```python
from build123d import *

# Parameters (mm, degrees)
SKETCH_1_W          = 23
SKETCH_1_H          = 10.8
EXTRUDE_1_DEPTH     = 34
CUT_EXTRUDE_1_DEPTH = 35
SKETCH_3_W          = 7
SKETCH_3_H          = 22
EXTRUDE_2_DEPTH     = 9
EXTRUDE_3_DEPTH     = 22
SKETCH_7_R          = 3.25
CUT_EXTRUDE_7_DEPTH = 1
CUT_EXTRUDE_8_REACH = 11.8
SKETCH_8_R          = 1.5


with BuildPart() as part:
    # 草图1 → 凸台-拉伸1 (new body)
    with BuildSketch(Plane(origin=(0, 0, 0), x_dir=(1, 0, 0), z_dir=(0, 1, 0))):
        Rectangle(SKETCH_1_W, SKETCH_1_H)
    extrude(amount=EXTRUDE_1_DEPTH)

    # 草图2 → 切除-拉伸1 (cut, through all)
    with BuildSketch(Plane(origin=(0, 34, 0), x_dir=(1, 0, 0), z_dir=(0, 1, 0))):
        Polygon((-6.5, 1.4), (6.5, 1.4), (6.5, -2.4), (3.15, -2.4), (3.15, -5.4), (-3.15, -5.4), (-3.15, -2.4), (-6.5, -2.4), align=None)
    extrude(amount=-CUT_EXTRUDE_1_DEPTH, mode=Mode.SUBTRACT)

    # 草图3 → 凸台-拉伸2 (add)
    with BuildSketch(Plane(origin=(0, 0, -5.4), x_dir=(-1, 0, 0), z_dir=(0, 0, -1))):
        with Locations((-10, 17)):
            Rectangle(SKETCH_3_W, SKETCH_3_H)
        with Locations((10, 17)):
            Rectangle(SKETCH_3_W, SKETCH_3_H)
    extrude(amount=-EXTRUDE_2_DEPTH)

    # 草图5 → 凸台-拉伸3 (add)
    with BuildSketch(Plane.XZ.offset(-6)):
        Polygon((11.5, 5.4), (11.5, 3.6), (13.5, 3.6), align=None)
        Polygon((-13.5, 3.6), (-11.5, 5.4), (-11.5, 3.6), align=None)
    extrude(amount=-EXTRUDE_3_DEPTH)

    # 草图7 → 切除-拉伸7 (cut)
    with BuildSketch(Plane.XY.offset(5.4)):
        with Locations((-10, 24.5)):
            Circle(SKETCH_7_R)
        with Locations((-10, 9.5)):
            Circle(SKETCH_7_R)
        with Locations((10, 9.5)):
            Circle(SKETCH_7_R)
        with Locations((10, 24.5)):
            Circle(SKETCH_7_R)
    extrude(amount=-CUT_EXTRUDE_7_DEPTH, mode=Mode.SUBTRACT)

    # 草图8 → 切除-拉伸8 (cut, up to next)
    with BuildSketch(Plane.XY.offset(4.4), mode=Mode.PRIVATE) as cut_extrude_8_sk1:
        with Locations((-10, 24.5)):
            Circle(SKETCH_8_R)
    cut_extrude_8_tool1 = extrude(cut_extrude_8_sk1.sketch, amount=-CUT_EXTRUDE_8_REACH, mode=Mode.PRIVATE) & part.part
    add(cut_extrude_8_tool1.solids().sort_by_distance((-10, 24.5, 4.4))[0], mode=Mode.SUBTRACT)
    # 草图8 → 切除-拉伸8 (cut, up to next)
    with BuildSketch(Plane.XY.offset(4.4), mode=Mode.PRIVATE) as cut_extrude_8_sk2:
        with Locations((10, 24.5)):
            Circle(SKETCH_8_R)
    cut_extrude_8_tool2 = extrude(cut_extrude_8_sk2.sketch, amount=-CUT_EXTRUDE_8_REACH, mode=Mode.PRIVATE) & part.part
    add(cut_extrude_8_tool2.solids().sort_by_distance((10, 24.5, 4.4))[0], mode=Mode.SUBTRACT)
    # 草图8 → 切除-拉伸8 (cut, up to next)
    with BuildSketch(Plane.XY.offset(4.4), mode=Mode.PRIVATE) as cut_extrude_8_sk3:
        with Locations((-10, 9.5)):
            Circle(SKETCH_8_R)
    cut_extrude_8_tool3 = extrude(cut_extrude_8_sk3.sketch, amount=-CUT_EXTRUDE_8_REACH, mode=Mode.PRIVATE) & part.part
    add(cut_extrude_8_tool3.solids().sort_by_distance((-10, 9.5, 4.4))[0], mode=Mode.SUBTRACT)
    # 草图8 → 切除-拉伸8 (cut, up to next)
    with BuildSketch(Plane.XY.offset(4.4), mode=Mode.PRIVATE) as cut_extrude_8_sk4:
        with Locations((10, 9.5)):
            Circle(SKETCH_8_R)
    cut_extrude_8_tool4 = extrude(cut_extrude_8_sk4.sketch, amount=-CUT_EXTRUDE_8_REACH, mode=Mode.PRIVATE) & part.part
    add(cut_extrude_8_tool4.solids().sort_by_distance((10, 9.5, 4.4))[0], mode=Mode.SUBTRACT)


solid = part.part
```
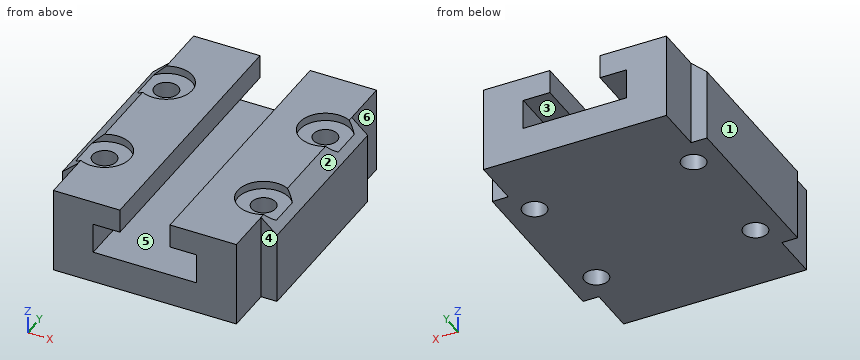
The listing builds one solid part. Answer for the finished solid, in the listing's coordinates (mm). Face numbers are marked on the shaded views. A direction names the side the tool comes from. Give positions to 0.01 mm unless a question says otherwise; leave off trailing zeros. Order: outer loops, then holes, each group sorted by start corner. A loop starts at its lowest first (then second) coordinate and runs counter-clockwise, first axis right, second up. Notation, with made-up numbers: (12.25, 1) -> (49.25, 1) arc R17 ccw to (49.25, 19) -> close; hole circle Ø8 at (32, 47.5). An arc over 180 degrees is marked (long way). Answer as a JSON object with one key per item and string values. Group by question number.
Item 1: The part is cut by section D-D on x = 5.75. Write down the section's boundary in (y, z).
Item 2: The part is cut by section B-B on z = -0.25. Write down the section's boundary in (x, y).
Item 3: Determine the mould class of the marked faces 1, 2 and 3 for opening direction Z: pulls with the +Z half, pulls with the -Z half, needs draft (parallel to the pull), parting line crosses it, or undercut.
Item 4: A tool of negligible diameter and unlimited length cuts with its end or side. For the marked faces 4, 5 and 6, from which of +Z, -Z, +X, -X, +Y, -Y can it reach the whole face along a straight path? Write none if from no direction.
Item 5: Flat-ended cylindrical pins translate along their axes: pin 1 (6.5 mm diameter, centred on x = -1.5, y = 9.5, fed in from +Z); pin 2 (4.5 mm diameter, centred on x = -10.5, y = 25, fed in from +Z); pin 3 (2.5 mm diameter, centred on x = 10, y = 24.5, fed in from +Z); pin 4 (1.8 mm diameter, centred on y = 1.5, z = 2.5, fed in from -X). Find the tip coordinate at first contact, or state that the pin passes through.
Item 6: The part is cut by section A-A on x = 10. Write down the section's boundary in (y, z), and give its area (3 significant figures).
Item 7: Consider L1, parallel to Y at x = -10, z = 5; L2, parallel to Y at x = -10, z = 2.75; L3, parallel to Z at x = -5.25, y = 26. Determine where each line is inside the solid, lowest interval first. Write a range as from..to.
Item 8: The part is cut by section C-C on y = 24.5. Write down the section's boundary in (x, z), and give its area (3 significant figures).
Result set:
{
 "1": {"outline": "(0, -5.4) -> (34, -5.4) -> (34, -1.4) -> (0, -1.4) -> close; (0, 2.4) -> (34, 2.4) -> (34, 5.4) -> (0, 5.4) -> close"},
 "2": {"outline": "(-13.5, 6) -> (-11.5, 6) -> (-11.5, 0) -> (-6.5, 0) -> (-6.5, 34) -> (-11.5, 34) -> (-11.5, 28) -> (-13.5, 28) -> close; (6.5, 0) -> (11.5, 0) -> (11.5, 6) -> (13.5, 6) -> (13.5, 28) -> (11.5, 28) -> (11.5, 34) -> (6.5, 34) -> close; hole circle Ø3 at (-10, 9.5); hole circle Ø3 at (-10, 24.5); hole circle Ø3 at (10, 9.5); hole circle Ø3 at (10, 24.5)"},
 "3": {"face 1": "needs draft", "face 2": "pulls with the +Z half", "face 3": "undercut"},
 "4": {"face 4": "+Z, -Z, +X, -Y", "face 5": "+Y, -Y", "face 6": "+Z, -Z, +X, +Y"},
 "5": {"pin 1": "z = 5.4", "pin 2": "z = 4.4", "pin 3": "through", "pin 4": "x = -11.5"},
 "6": {"outline": "(0, -5.4) -> (8, -5.4) -> (8, 4.4) -> (6.25, 4.4) -> (6.25, 5.4) -> (0, 5.4) -> close; (11, -5.4) -> (23, -5.4) -> (23, 4.4) -> (21.25, 4.4) -> (21.25, 5.4) -> (12.75, 5.4) -> (12.75, 4.4) -> (11, 4.4) -> close; (26, -5.4) -> (34, -5.4) -> (34, 5.4) -> (27.75, 5.4) -> (27.75, 4.4) -> (26, 4.4) -> close", "area": "295 mm²"},
 "7": {"L1": "0..6.25, 12.75..21.25, 27.75..34", "L2": "0..8, 11..23, 26..34", "L3": "-5.4..-1.4, 2.4..5.4"},
 "8": {"outline": "(-13.5, -5.4) -> (-11.5, -5.4) -> (-11.5, 4.4) -> (-12.61, 4.4) -> (-13.5, 3.6) -> close; (-8.5, -5.4) -> (8.5, -5.4) -> (8.5, 4.4) -> (6.75, 4.4) -> (6.75, 5.4) -> (3.15, 5.4) -> (3.15, 2.4) -> (6.5, 2.4) -> (6.5, -1.4) -> (-6.5, -1.4) -> (-6.5, 2.4) -> (-3.15, 2.4) -> (-3.15, 5.4) -> (-6.75, 5.4) -> (-6.75, 4.4) -> (-8.5, 4.4) -> close; (11.5, -5.4) -> (13.5, -5.4) -> (13.5, 3.6) -> (12.61, 4.4) -> (11.5, 4.4) -> close", "area": "150 mm²"}
}
